The drawing under review shows one solid part. Ordinate dimensions are in mm from its lowest x, y, z. A direction names the side the tool comes from. Coordinates: 2 decimals unless noted, no trailing zeros. Order: outer loops, then holes, each group sorted by start corner. A loop starts at its lowest first (then second) coordinate and runs counter-clockwise, first axis right, second up.
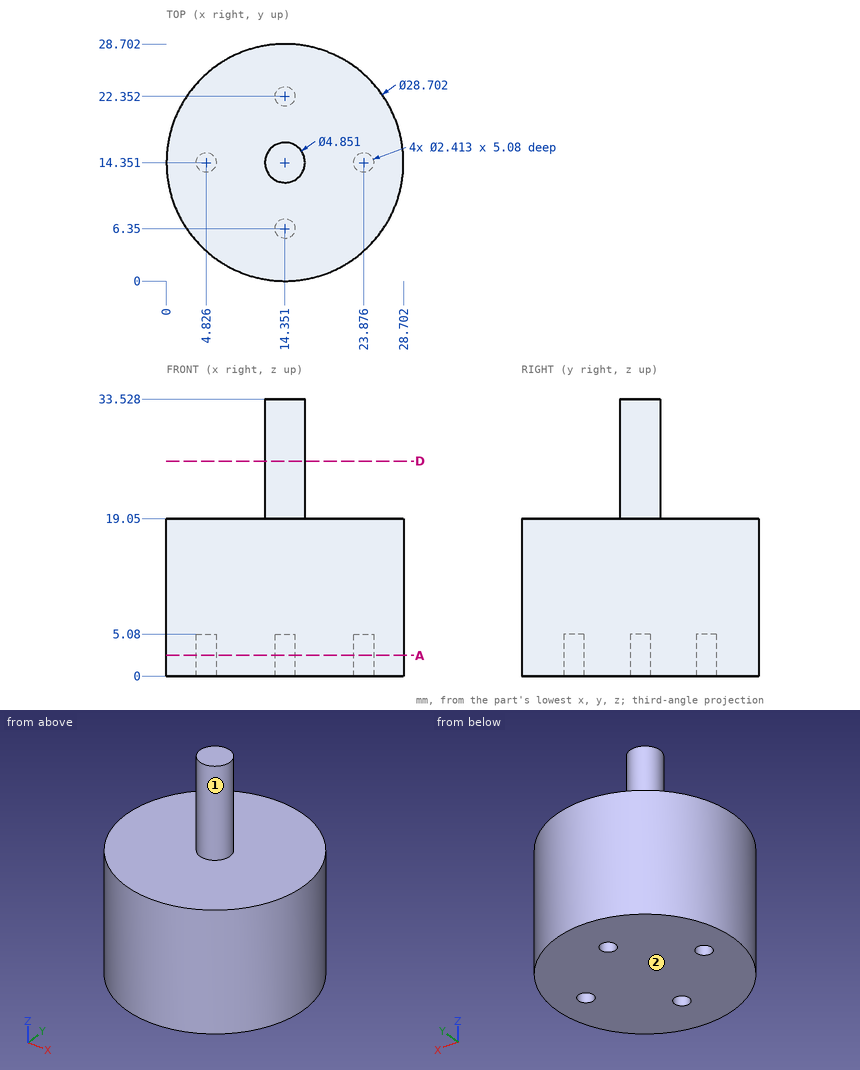
1. Machinability: for the marked faces 1 and 2, which of the approach directions +Z, -Z, +X, -X, +Y, -Y give a long, thin tool a straight path to every point of the face, cutting with its end or side? Answer none if there is none.
Answer below:
face 1: +Z
face 2: -Z, +X, -X, +Y, -Y
2. To check wall thickness, follow L1, parallel to Z at x = 6, y = 24.25; L2, parallel to X at y = 14.5, z = 28.5; L3, parallel to Z at x = 14.75, y = 22.75. State the ranges of each line that lie inside material, in increasing order.
Answer below:
L1: z = 0 to 19.05
L2: x = 11.93 to 16.77
L3: z = 5.08 to 19.05
3. Take a section at A-A, the plane z = 2.5. Give the number of separate pieces and of enclosed holes in the cut face, plus the area to 3 significant figures.
Answer below:
separate pieces: 1
enclosed holes: 4
area: 629 mm2
4. Take a section at D-D, the plane z = 26. Give the boundary of the cut face in (x, y) (1 decimal).
Answer below:
outline: circle Ø4.9 at (14.4, 14.4)
5. Clearance check with flat-ended pins moving along their axes: pin 1 Ø1.5 at (y, z) = (8, 14) entering from +X; pin 2 Ø8 at (x, y) = (21.5, 12) entering from -Z; pin 3 Ø1.5 at (y, z) = (6, 13) entering from -X; pin 4 Ø1.9 at (x, y) = (4.826, 14.351) entering from -Z. State where each tip first meets the part, or that it passes through.
Answer below:
pin 1: stops at x = 27.56
pin 2: stops at z = 0
pin 3: stops at x = 2.18
pin 4: stops at z = 5.08
